Geometry check sheet. Reference: drawing and pictorial views, mm from the part's lowest x, y, z. A direction names the side the tool comes from. Give positions to 0.01 mm unless a question says otherwise; leave off trailing zeros. Write each loop counter-clockwise with the first axis right and the second up, starting at its lowest first coordinate (ties: lowest second). Pieces come first, ordered by that corner, then holes. Notation, with made-up numbers: (-19.75, 34) - (15.25, 34) arc R23 cw to (15.25, 59) - close; hole circle Ø5 at (19.25, 41). An arc over 180 degrees is marked (long way). Put each result on its own line as item: value.
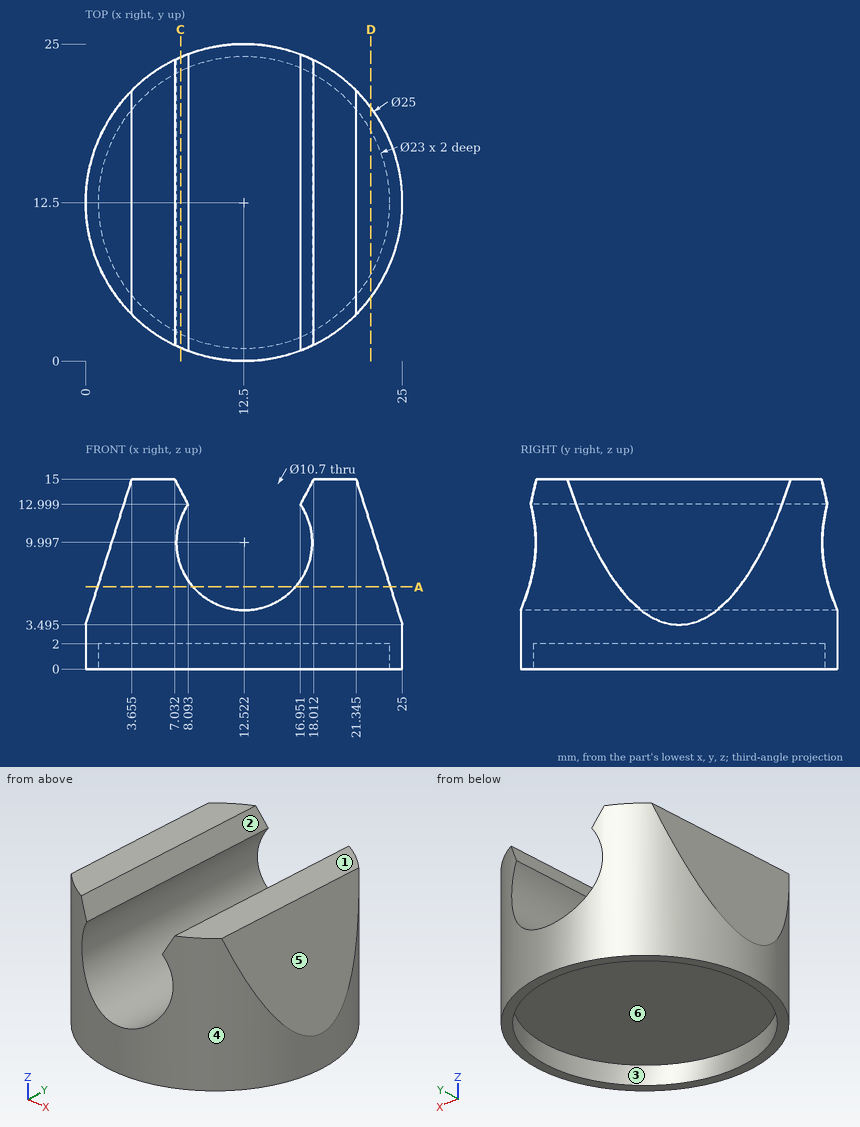
Q1. Section check D-D, the plane x = 22.5. Record the cut outline in (y, z) (1 decimal).
Answers follow:
outline: (5, 0) - (6.8, 0) - (6.8, 2) - (18.2, 2) - (18.2, 0) - (20, 0) - (20, 11.4) - (5, 11.4) - close
Q2. Go/stop test with flat-tipped pins: pin 1 Ø3 at (y, z) = (7.5, 9) entering from +X; pin 2 Ø10 at (x, y) = (17.5, 17) entering from +Z; pin 3 Ø8 at (y, z) = (4.5, 2) entering from +X; pin 4 Ø1.5 at (y, z) = (9.5, 4) entering from +X. Record where each tip stops, or that it passes through.
Answers follow:
pin 1: stops at x = 23.73
pin 2: stops at z = 15
pin 3: stops at x = 24.34
pin 4: stops at x = 24.8
Q3. Set-up check for the marked faces 1 and 2: record each of +Z, -Z, +X, -X, +Y, -Y from which the full face is reachable in a straight line by a thin tool's end or side.
Answers follow:
face 1: +Z, +X, -X, +Y, -Y
face 2: +Z, +Y, -Y
Q4. Section check A-A, the plane z = 6.5. Record the cut outline in (x, y) (1 decimal), plus the area to 3 significant figures.
Answers follow:
outline: (1, 7.7) arc R12.5 ccw to (8.5, 0.7) - (8.5, 24.3) arc R12.5 ccw to (1, 17.3) - close; (16.6, 0.7) arc R12.5 ccw to (24, 7.7) - (24, 17.3) arc R12.5 ccw to (16.6, 24.3) - close
area: 280 mm2
Q5. Release check for a two-part mould opening along X. For the marked faces 3, 4, 5 and 6 record: released by +X, released by -X, zero draft, split by the parting line, or undercut.
Answers follow:
face 3: undercut
face 4: split by the parting line
face 5: released by +X
face 6: undercut
Q6. Section check C-C, the plane x = 7.5. Record the cut outline in (y, z).
Answers follow:
outline: (1.04, 0) - (2.14, 0) - (2.14, 2) - (22.86, 2) - (22.86, 0) - (23.96, 0) - (23.96, 8.15) - (1.04, 8.15) - close; (1.04, 11.84) - (23.96, 11.84) - (23.96, 14.12) - (1.04, 14.12) - close
Q7. Scan lines: line 1 along Y through (x, z) = (12.5, 1.1); line 2 along X through (y, z) = (17.5, 10.25) (1 decimal); line 3 along X through (y, z) = (13, 11.25). Record each from-to range of solid material in increasing order.
Answers follow:
line 1: y = 0 to 1, 24 to 25
line 2: x = 2.1 to 7.2, 17.9 to 22.9
line 3: x = 2.46 to 7.32, 17.72 to 22.54
